Build history of the part. All positions in model axes, mm. Face numbers are marked on the shaded views. Round coordinates to 2 decimals unless told otherwise and drop trailing zeros. Write each loop counter-clockwise with the first axis right and the second up, starting at its lowest first coordinate (ties: lowest second). Pieces come first, ordered by that corner, then holes.
from build123d import *

# Parameters (mm, degrees)
CROQUIS1_W              = 50.8
CROQUIS1_H              = 80
SALIENTE_EXTRUIR1_DEPTH = 6.35
CROQUIS4_R              = 2
CORTAR_EXTRUIR3_DEPTH   = 48.806720239
CROQUIS5_W              = 50.8
CROQUIS5_H              = 12.7
CORTAR_EXTRUIR4_DEPTH   = 48.806720239
CROQUIS6_W              = 50.8
CROQUIS6_H              = 20.526572449
CORTAR_EXTRUIR5_DEPTH   = 10
CROQUIS7_W              = 50.8
CROQUIS7_H              = 6.773427551
CORTAR_EXTRUIR6_DEPTH   = 10
CROQUIS9_R              = 5
CORTAR_EXTRUIR7_DEPTH   = 10


with BuildPart() as part:
    # Croquis1 → Saliente-Extruir1 (new body)
    with BuildSketch(Plane(origin=(0, 0, 0), x_dir=(1, 0, 0), z_dir=(0, 1, 0))):
        Rectangle(CROQUIS1_W, CROQUIS1_H)
    extrude(amount=SALIENTE_EXTRUIR1_DEPTH)

    # Croquis4 → Cortar-Extruir3 (cut, through all)
    with BuildSketch(Plane(origin=(0, 6.35, 0), x_dir=(1, 0, 0), z_dir=(0, 1, 0))):
        with Locations(Location((-19, 19.466091849, 0), (0, 0, 270))):
            Circle(CROQUIS4_R)
        with Locations(Location((19, 19.466091849, 0), (0, 0, 270))):
            Circle(CROQUIS4_R)
        with Locations(Location((0, 0.466091849, 0), (0, 0, 270))):
            Circle(CROQUIS4_R)
    extrude(amount=-CORTAR_EXTRUIR3_DEPTH, mode=Mode.SUBTRACT)

    # Croquis5 → Cortar-Extruir4 (cut, through all)
    with BuildSketch(Plane(origin=(0, 6.35, 0), x_dir=(1, 0, 0), z_dir=(0, 1, 0))):
        with Locations((0, -33.65)):
            Rectangle(CROQUIS5_W, CROQUIS5_H)
    extrude(amount=-CORTAR_EXTRUIR4_DEPTH, mode=Mode.SUBTRACT)

    # Croquis6 → Cortar-Extruir5 (cut)
    with BuildSketch(Plane(origin=(0, 6.35, 0), x_dir=(1, 0, 0), z_dir=(0, 1, 0))):
        with Locations((0, -17.036713776)):
            Rectangle(CROQUIS6_W, CROQUIS6_H)
    extrude(amount=-CORTAR_EXTRUIR5_DEPTH, mode=Mode.SUBTRACT)

    # Croquis7 → Cortar-Extruir6 (cut)
    with BuildSketch(Plane.XZ):
        with Locations((0, -36.613286225)):
            Rectangle(CROQUIS7_W, CROQUIS7_H)
    extrude(amount=-CORTAR_EXTRUIR6_DEPTH, mode=Mode.SUBTRACT)

    # Croquis9 → Cortar-Extruir7 (cut)
    with BuildSketch(Plane.XZ):
        with Locations(Location((0, -19.466091849, 0), (0, 0, 270))):
            Circle(CROQUIS9_R)
    extrude(amount=-CORTAR_EXTRUIR7_DEPTH, mode=Mode.SUBTRACT)


solid = part.part
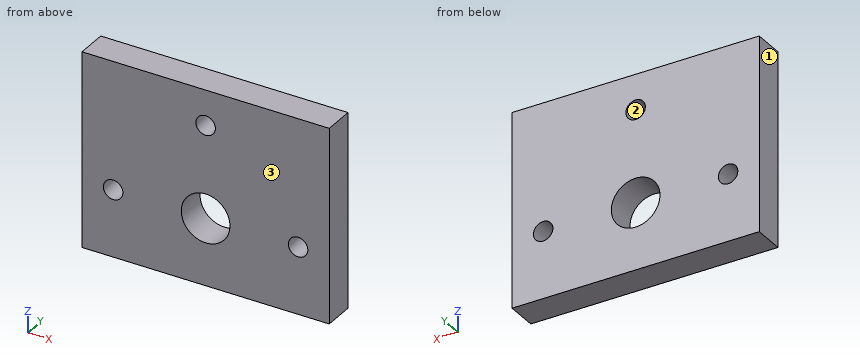
1) Mould opens along X. For the marked faces 1, 2 and 3 say: released by +X, released by -X, zero draft, split by the parting line, or undercut.
Results:
face 1: released by -X
face 2: undercut
face 3: zero draft
2) Wall check: L1, parallel to X at y = 1, z = 0.5; L2, parallel to Z at x = 4, y = 4; L3, parallel to X at y = 3.25, z = -21.5. Give the ranges that are in metal, low to high.
Results:
L1: x = -25.4 to -1.75, 1.75 to 25.4
L2: z = -33.23 to -22.47, -16.47 to 6.77
L3: x = -25.4 to -4.57, 4.57 to 25.4
3) Slice it at B-B (x = 0). Write the cut outline in (y, z), plus the area to 3 significant figures.
Results:
outline: (0, -33.23) - (6.35, -33.23) - (6.35, -24.47) - (0, -24.47) - close; (0, -14.47) - (6.35, -14.47) - (6.35, -2.47) - (0, -2.47) - close; (0, 1.53) - (6.35, 1.53) - (6.35, 6.77) - (0, 6.77) - close
area: 165 mm2
4) Slice it at A-A (x = -19). Write the cut outline in (y, z).
Results:
outline: (0, -33.23) - (6.35, -33.23) - (6.35, -21.47) - (0, -21.47) - close; (0, -17.47) - (6.35, -17.47) - (6.35, 6.77) - (0, 6.77) - close
5) Slice it at D-D (y = 1). Write the cut outline in (x, z).
Results:
outline: (-25.4, -33.23) - (25.4, -33.23) - (25.4, 6.77) - (-25.4, 6.77) - close; hole circle Ø4 at (-19, -19.47); hole circle Ø10 at (0, -19.47); hole circle Ø4 at (0, -0.47); hole circle Ø4 at (19, -19.47)
6) Slice it at C-C (z = -16). Write the cut outline in (x, y), plus the area to 3 significant figures.
Results:
outline: (-25.4, 0) - (-3.6, 0) - (-3.6, 6.35) - (-25.4, 6.35) - close; (3.6, 0) - (25.4, 0) - (25.4, 6.35) - (3.6, 6.35) - close
area: 277 mm2
